```python
from build123d import *

# Parameters (mm, degrees)
SKETCH1_W           = 12
SKETCH1_H           = 13
SKETCH1_W_2         = 9.6
SKETCH1_H_2         = 10.6
BOSS_EXTRUDE1_DEPTH = 10
SKETCH2_W           = 4.5
SKETCH2_H           = 13
BOSS_EXTRUDE2_DEPTH = 1
SKETCH3_W           = 9.6
SKETCH3_H           = 1.2
CUT_EXTRUDE1_DEPTH  = 7


with BuildPart() as part:
    # Sketch1 → Boss-Extrude1 (new body)
    with BuildSketch(Plane(origin=(0, 0, 0), x_dir=(1, 0, 0), z_dir=(0, 1, 0))):
        Rectangle(SKETCH1_W, SKETCH1_H)
        Rectangle(SKETCH1_W_2, SKETCH1_H_2, mode=Mode.SUBTRACT)
    extrude(amount=BOSS_EXTRUDE1_DEPTH)

    # Sketch2 → Boss-Extrude2 (add)
    with BuildSketch(Plane(origin=(0, 0, 0), x_dir=(1, 0, 0), z_dir=(0, 1, 0))):
        with Locations((-8.25, 0)):
            Rectangle(SKETCH2_W, SKETCH2_H)
        with Locations((8.25, 0)):
            Rectangle(SKETCH2_W, SKETCH2_H)
    extrude(amount=BOSS_EXTRUDE2_DEPTH)

    # Sketch3 → Cut-Extrude1 (cut)
    with BuildSketch(Plane(origin=(0, 10, 0), x_dir=(1, 0, 0), z_dir=(0, 1, 0))):
        with Locations((0, 5.9)):
            Rectangle(SKETCH3_W, SKETCH3_H)
    extrude(amount=-CUT_EXTRUDE1_DEPTH, mode=Mode.SUBTRACT)


solid = part.part
```
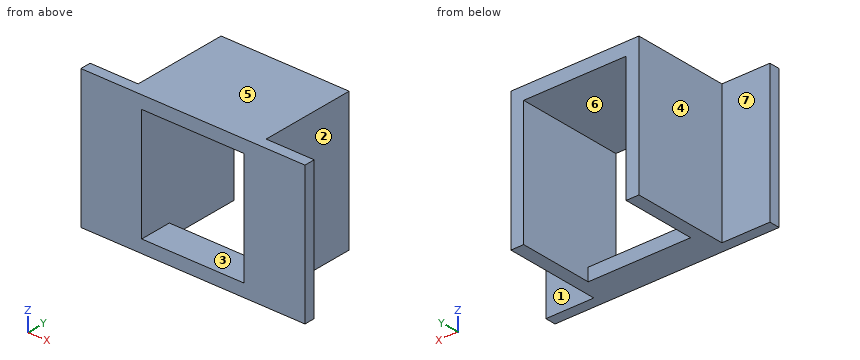
The listing builds one solid part. Answer for the finished solid, in the listing's coordinates (mm). Face numbers are marked on the shaded views. A direction names the side the tool comes from. Give positions to 0.01 mm unless a question says otherwise; leave off trailing zeros. Write each loop counter-clockwise with the first axis right and the second up, starting at its lowest first coordinate (ties: lowest second). Pieces come first, ordered by that corner, then holes. Notation, with made-up numbers: (-25.5, 32) -> (1.5, 32) arc R23 cw to (1.5, 52) -> close; hole circle Ø2 at (44, 63.25). An arc over 180 degrees is marked (long way). Write item = value, one per line. Start each with the question number.
1) Which of the six approach directions +Z, -Z, +X, -X, +Y, -Y give full straight-line access (tool end or side, diameter ignored) to the marked faces 5, 6 and 7?
2) Each of these flat-tipped pins is pushed along its axis until it touches: pin 1 (4.5 mm diameter, centred on y = 6.5, z = -2.5, fed in from +X); pin 2 (2 mm diameter, centred on y = 7, z = 1.5, fed in from -X); pin 3 (1.3 mm diameter, centred on x = -9.5, z = -1, fed in from +Y). Where does it stop, or does it pass through?
3) The part is cut by section D-D, the plane y = 8.5. Determine the outline of the cut face in (x, z).
4) Straight lines are drawn through the part: line 1 along Z through (x, y) = (3, 2.75); line 2 along X through (y, z) = (2, -0.75); line 3 along Y through (x, z) = (8.25, 2.25). For each, find the intervals that lie inside material, in ascending order.
5) Determine the mould class of the marked faces 1, 2, 3 and 4 for opening direction X: +X half, -X half, draft (parallel to the pull), parting line (faces both ways), or undercut.
6) The part is cut by section A-A, the plane x = -0.5. Determine the outline of the cut face in (y, z), and give its area (3 significant figures).
7) The part is cut by section C-C, the plane y = 2. Determine the outline of the cut face in (x, z).
8) The part is cut by section B-B, the plane z = -0.5. Determine the outline of the cut face in (x, y).
Solutions:
q1.face_5 = +Z, +X, -X, +Y, -Y
q1.face_6 = +Y, -Y
q1.face_7 = +Z, -Z, -X, +Y
q2.pin_1 = 6
q2.pin_2 = -6
q2.pin_3 = 1
q3.outline = (-6, -6.5) -> (-4.8, -6.5) -> (-4.8, 5.3) -> (4.8, 5.3) -> (4.8, -6.5) -> (6, -6.5) -> (6, 6.5) -> (-6, 6.5) -> close
q4.line_1 = -6.5 to -5.3, 5.3 to 6.5
q4.line_2 = -6 to -4.8, 4.8 to 6
q4.line_3 = 0 to 1
q5.face_1 = draft
q5.face_2 = +X half
q5.face_3 = undercut
q5.face_4 = -X half
q6.outline = (0, -6.5) -> (3, -6.5) -> (3, -5.3) -> (0, -5.3) -> close; (0, 5.3) -> (10, 5.3) -> (10, 6.5) -> (0, 6.5) -> close
q6.area = 15.6 mm²
q7.outline = (-6, -6.5) -> (6, -6.5) -> (6, 6.5) -> (-6, 6.5) -> close; hole (-4.8, -5.3) -> (4.8, -5.3) -> (4.8, 5.3) -> (-4.8, 5.3) -> close
q8.outline = (-10.5, 0) -> (-4.8, 0) -> (-4.8, 10) -> (-6, 10) -> (-6, 1) -> (-10.5, 1) -> close; (4.8, 0) -> (10.5, 0) -> (10.5, 1) -> (6, 1) -> (6, 10) -> (4.8, 10) -> close
